Source: CAD feature listing. Evaluate the final solid. Frame: model axes, mm. Round coordinates to 2 decimals unless told otherwise and drop trailing zeros. Write each loop counter-clockwise with the first axis right and the second up, starting at its lowest first coordinate (ties: lowest second). Pieces come first, ordered by that corner, then holes. Notation, with made-up numbers: M -0.5,16 L 7.5,16 A12 cw 7.5,26 Z; hole C 17,38 d2. An arc over 180 degrees is marked long. Answer in a Markdown table with one row per item.
from build123d import *

# Parameters (mm, degrees)
F0_R     = 246.0625
F0_R_2   = 16.0248299709
F1_DEPTH = 4.7625
F2_DEPTH = 4.7752
F4_D     = 6.35
F6_DEPTH = 9.5387
F8_D     = 6.35


with BuildPart() as f1:
    # F0 (on Front) → F1 (new body)
    with BuildSketch(Plane.XZ):
        Circle(F0_R)
        Circle(F0_R_2, mode=Mode.SUBTRACT)
    extrude(amount=F1_DEPTH)

    # F2 (add): a face of the model
    f2_faces = [f1.faces().sort_by_distance(p)[0] for p in [
        (-239.1028015062, -4.7625, 0),
    ]]
    extrude(f2_faces, amount=F2_DEPTH)

    # F4 (through all)
    with Locations(Plane(origin=(0, 0, 0), x_dir=(1, 0, 0), z_dir=(0, 1, 0))):
        with Locations((23.3807638288, -5.0180926919), (28.036672622, 0), (33.8565558195, -5.3090867586), (38.5124646127, 0), (43.1683734059, -5.3090867586), (48.1152758002, 0), (57.7180869877, 0), (62.6649931073, -5.0180926919), (67.611888051, 0), (73.7227723002, -5.0180926919), (53.0621781945, -5.0180926919), (80.415636301, 0)):
            Hole(F4_D / 2)

    # F5 (on Front) → F6 (cut, through all)
    with BuildSketch(Plane.XZ):
        with BuildLine():
            add(Edge.make_bspline(
                [(14.4555894658, 9.5869684592), (12.7334762365, 16.9557761401), (-4.4353525154, 19.925462082), (-8.1386631355, 16.0679295659)],
                knots=[0, 0, 0, 0, 23.5053846486, 23.5053846486, 23.5053846486, 23.5053846486], degree=3))
            Line((14.4555894658, 9.5869684592), (28.8158967792, 21.0863542243))
            add(Edge.make_bspline(
                [(28.8158967792, 21.0863542243), (22.4603216629, 32.5071383268), (-6.1850600177, 42.7067335695), (-17.1682926589, 31.9189709392)],
                knots=[0, 0, 0, 0, 47.2428964307, 47.2428964307, 47.2428964307, 47.2428964307], degree=3))
            Line((-17.1682926589, 31.9189709392), (-8.1386631355, 16.0679295659))
        make_face()
    extrude(amount=F6_DEPTH, mode=Mode.SUBTRACT)

    # F8 (through all)
    with Locations(Plane(origin=(0, 0, 0), x_dir=(1, 0, 0), z_dir=(0, 1, 0))):
        with Locations((226.2086173164, 0)):
            Hole(F8_D / 2)


solid = f1.part
Q1. Section D-D (x = -109). Return loops of the section in (y, z), and give its area (3 significant figures).
Solutions:
| item | result |
|---|---|
| outline | M -9.54,-220.6 L 0,-220.6 L 0,220.6 L -9.54,220.6 Z |
| area | 4,210 mm2 |
Q2. Section A-A (x = 0). State how many separate pieces and enclosed holes the cut face has, and give its area (3 significant figures).
Solutions:
| item | result |
|---|---|
| separate pieces | 3 |
| enclosed holes | 0 |
| area | 4,210 mm2 |
Q3. Pull-direction query (X, two-part tool) for faces 1 (the flat face through (-3, 0, -51)), 2 (the cylindrical face through (-53.34, -4.7, -240.21)), 3 (the flat face through (21.54, -4.7, 15.26)); classes: pulls with the +X half, pulls with the -X half, needs draft (parallel to the pull), parting line crosses it, or undercut.
Solutions:
| item | result |
|---|---|
| face 1 | needs draft |
| face 2 | parting line crosses it |
| face 3 | undercut |
Q4. Contact query for flat-ended pins moving along their axis: pin 1 Ø1.5 at (y, z) = (-4.5, -105.5) entering from -X; pin 2 Ø8.5 at (x, z) = (226.21, 0) entering from -Y; pin 3 Ø1.5 at (x, y) = (-12, -5.5) entering from +Z; pin 4 Ø5 at (x, y) = (95, -6) entering from -Z. Output: stop coordinate, or through.
Solutions:
| item | result |
|---|---|
| pin 1 | stops at x = -222.65 |
| pin 2 | stops at y = -9.54 |
| pin 3 | stops at z = 245.81 |
| pin 4 | stops at z = -228.01 |
Q5. Material intervals for probe 1 along Z at (x, y) = (6.5, -0.25); probe 2 along Z at (x, y) = (10.5, -4); probe 3 along Z at (x, y) = (29, -3), sorted ascending.
Solutions:
| item | result |
|---|---|
| probe 1 | z = -245.98 to -14.65, 14.65 to 16.28, 35.12 to 245.98 |
| probe 2 | z = -245.84 to -12.11, 12.11 to 14.39, 33.9 to 245.84 |
| probe 3 | z = -244.35 to -3.03, 3.03 to 244.35 |
Q6. Section B-B (z = -174). Return loops of the section in (x, y).
Solutions:
| item | result |
|---|---|
| outline | M -173.98,-9.54 L 173.98,-9.54 L 173.98,0 L -173.98,0 Z |
